The model under review builds one solid part; all positions refer to its coordinate system, in mm. A direction names the side the tool comes from. Coordinates: 2 decimals unless noted, no trailing zeros. Order: outer loops, then holes, each group sorted by start corner. A loop starts at its lowest first (then second) coordinate and runs counter-clockwise, first axis right, second up. Notation, with made-up numbers: M 48,40 L 74,40 A13 ccw 74,55 Z; hole C 78.25,-29 d9. An arc over 180 degrees is marked long. One line per item, written item: value.
```python
from build123d import *

# Parameters (mm, degrees)
SKETCH1_W                = 44.45
SKETCH1_H                = 44.45
SKETCH1_W_2              = 38.1
SKETCH1_H_2              = 38.1
BOSS_EXTRUDE1_DEPTH      = 95.25
BOSS_EXTRUDE1_DEPTH_BACK = 95.25


with BuildPart() as part:
    # Sketch1 → Boss-Extrude1 (new body, two sides)
    with BuildSketch(Plane(origin=(0, 0, 0), x_dir=(1, 0, 0), z_dir=(0, 1, 0))) as boss_extrude1_sk:
        Rectangle(SKETCH1_W, SKETCH1_H)
        Rectangle(SKETCH1_W_2, SKETCH1_H_2, mode=Mode.SUBTRACT)
    extrude(amount=BOSS_EXTRUDE1_DEPTH)
    extrude(boss_extrude1_sk.sketch, amount=-BOSS_EXTRUDE1_DEPTH_BACK)


solid = part.part
```
(1) We need section B-B, the plane x = 11.5. State the section outline as (y, z) points (3 decimals).
Geometry results:
outline: M -95.25,-22.225 L 95.25,-22.225 L 95.25,-19.05 L -95.25,-19.05 Z; M -95.25,19.05 L 95.25,19.05 L 95.25,22.225 L -95.25,22.225 Z
(2) Mouldability with a two-part tool opening along Z and no side actions: class faces 1 (the flat face through (0, 1, -22.225)), 2 (the flat face through (19.4, 95.25, -0.3)), 3 (the flat face through (-19.05, 1, 0)) as +Z half, -Z half, draft (parallel to the pull), parting line (faces both ways), or undercut.
Geometry results:
face 1: -Z half
face 2: draft
face 3: undercut
(3) For L1, parallel to X at y = -82.5, z = -1 (3 decimals), list the stretches that pass through material, from the lowest coordinate up.
Geometry results:
L1: x = -22.225 to -19.05, 19.05 to 22.225
(4) Tool access review of faces 4 (the flat face through (0, 1, 19.05)), 5 (the flat face through (-22.225, 1, 0)): name each direction out of +Z, -Z, +X, -X, +Y, -Y from which nothing blocks a thin tool from reaching the whole face with its end or side.
Geometry results:
face 4: +Y, -Y
face 5: +Z, -Z, -X, +Y, -Y
(5) We need section C-C, the plane y = -47. State the section outline as (x, z) points (3 decimals).
Geometry results:
outline: M -22.225,-22.225 L 22.225,-22.225 L 22.225,22.225 L -22.225,22.225 Z; hole M -19.05,-19.05 L 19.05,-19.05 L 19.05,19.05 L -19.05,19.05 Z
(6) Insertion check: pin 1 Ø12 at (x, z) = (-9, -6.5) entering from +Y. The pin has a flat end and moves straight along its axis. Give the tip position at first contact, or say it passes through.
Geometry results:
pin 1: passes through
(7) We need section A-A, the plane z = 13.5. State the section outline as (x, y) points (3 decimals).
Geometry results:
outline: M -22.225,-95.25 L -19.05,-95.25 L -19.05,95.25 L -22.225,95.25 Z; M 19.05,-95.25 L 22.225,-95.25 L 22.225,95.25 L 19.05,95.25 Z
